For this review, take the finished solid that the model builds, in its own axes (mm). Face numbers are marked on the shaded views. Coordinates: 2 decimals unless noted, no trailing zeros. Write each loop counter-clockwise with the first axis right and the second up, starting at its lowest first coordinate (ties: lowest second). Pieces come first, ordered by that corner, then holes. Notation, with made-up numbers: (48, 51.25) -> (76, 51.25) arc R21 ccw to (76, 67.25) -> close; hole circle Ø3 at (-29, 24). An arc over 180 degrees is marked (long way). Put each result on its own line as item: value. Start each with the question number.
Item 1: To check wall thickness, follow L1, parallel to Y at x = 0, z = -4.45; L2, parallel to X at y = -0.5, z = -2.5; L3, parallel to Y at x = 2.25, z = -2.25. State the ranges of each line that lie inside material, in increasing order.
Item 2: Consider section A-A on z = 4.25. Give the boundary of the cut face in (x, y).
Item 3: The part is to be moulded in two halves that separate along Y. For the marked faces 1, 2 and 3, say which applies: +Y half, -Y half, draft (parallel to the pull), parting line (faces both ways), or undercut.
Item 4: Insertion check: P1, Ø1, axis at y = 1.5, z = -4.5, coming from the -X side; P2, Ø3, axis at x = 0, y = -3.5, coming from the +Z side; P3, Ø3, axis at x = -6, z = -2, coming from the +Y side; P4, Ø6, axis at x = 1, y = -2.5, coming from the -Z side. Each pin has a flat end and moves straight along its axis. Give the tip position at first contact, or say it passes through.
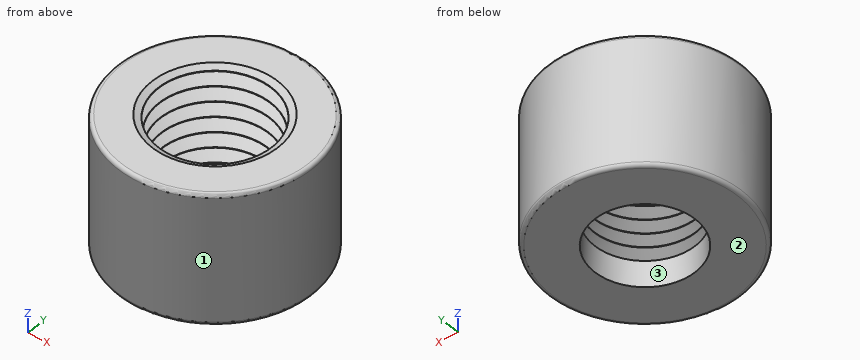
```python
from build123d import *

# Parameters (mm, degrees)
SKETCH1_R      = 9.398
EXTRUDE1_DEPTH = 6.35
SKETCH5_W      = 12.7
SKETCH5_H      = 4.869399387
FILLET1_R      = 0.352777778


with BuildPart() as part:
    # Sketch1 → Extrude1 (new body, symmetric)
    with BuildSketch(Plane.XY):
        Circle(SKETCH1_R)
    extrude(amount=EXTRUDE1_DEPTH, both=True)

    # Sketch5 → Cut-Revolve7 (revolve, cut)
    with BuildSketch(Plane(origin=(0, 0, 0), x_dir=(0, 0, -1), z_dir=(1, 0, 0))):
        with Locations((0, 2.434699694)):
            Rectangle(SKETCH5_W, SKETCH5_H)
    revolve(axis=Axis((0, 0, 0), (0, 0, -1)), mode=Mode.SUBTRACT)

    # Fillet1
    fillet1_edges = [part.edges().sort_by_distance(p)[0] for p in [
        (-9.398, 0, -6.35),
        (-9.398, 0, 6.35),
    ]]
    fillet(fillet1_edges, radius=FILLET1_R)

    # Sketch2 → Cut-Revolve5 (revolve, cut)
    with BuildSketch(Plane(origin=(0, 0, 0), x_dir=(0, 0, -1), z_dir=(1, 0, 0))):
        Polygon((-22.120436281, 7.622813225), (-21.540434076, 6.455429709), (-21.486747793, 6.452070868), (-20.765765115, 7.53805927), (-20.712078832, 7.534700429), (-20.132076627, 6.367316913), (-20.078390344, 6.363958072), (-19.357407666, 7.449946474), (-19.303721383, 7.446587633), (-18.723719178, 6.279204117), (-18.670032896, 6.275845277), (-17.949050217, 7.361833678), (-17.895363935, 7.358474838), (-17.31536173, 6.191091322), (-17.261675447, 6.187732481), (-16.540692769, 7.273720883), (-16.487006486, 7.270362042), (-15.907004281, 6.102978526), (-15.853317998, 6.099619685), (-15.13233532, 7.185608087), (-15.078649037, 7.182249246), (-14.498646832, 6.01486573), (-14.44496055, 6.01150689), (-13.723977871, 7.097495291), (-13.670291589, 7.094136451), (-13.090289384, 5.926752935), (-13.036603101, 5.923394094), (-12.315620423, 7.009382496), (-12.26193414, 7.006023655), (-11.681931935, 5.838640139), (-11.628245652, 5.835281298), (-10.907262974, 6.9212697), (-10.853576692, 6.917910859), (-10.273574486, 5.750527343), (-10.219888204, 5.747168503), (-9.498905526, 6.833156904), (-9.445219243, 6.829798064), (-8.865217038, 5.662414548), (-8.811530755, 5.659055707), (-8.090548077, 6.745044109), (-8.036861794, 6.741685268), (-7.456859589, 5.574301752), (-7.403173306, 5.570942911), (-6.682190628, 6.656931313), (-6.628504346, 6.653572472), (-6.04850214, 5.486188956), (-5.994815858, 5.482830116), (-5.27383318, 6.568818517), (-5.220146897, 6.565459677), (-4.640144692, 5.398076161), (-4.586458409, 5.39471732), (-3.865475731, 6.480705722), (-3.811789448, 6.477346881), (-3.231787243, 5.309963365), (-3.178100961, 5.306604524), (-2.457118282, 6.392592926), (-2.403432, 6.389234085), (-1.823429795, 5.221850569), (-1.769743512, 5.218491729), (-1.048760834, 6.30448013), (-0.995074551, 6.30112129), (-0.415072346, 5.133737774), (-0.361386063, 5.130378933), (0.359596615, 6.216367335), (0.413282898, 6.213008494), (0.993285103, 5.045624978), (1.046971385, 5.042266137), (1.767954064, 6.128254539), (1.821640346, 6.124895698), (2.401642551, 4.957512182), (2.455328834, 4.954153342), (3.176311512, 6.040141743), (3.229997795, 6.036782903), (3.81, 4.869399387), (3.81, 0), (-23.582480012, 0), (-23.582480012, 7.714284861), (-23.528793729, 7.71092602), (-22.948791524, 6.543542504), (-22.895105242, 6.540183664), (-22.174122563, 7.626172065), align=None)
    revolve(axis=Axis((0, 0, -97.9740637), (0, 0, 1)), mode=Mode.SUBTRACT)


solid = part.part
```
Return value:
1. L1: -9.4 to -4.87, 4.87 to 9.4
1. L2: -9.38 to -5, 5 to 9.38
1. L3: -9.12 to -4.76, 4.76 to 9.12
2. outline: circle Ø18.8 at (0, 0); hole circle Ø11.8 at (0, 0)
3. face 1: parting line
3. face 2: draft
3. face 3: undercut
4. P1: x = -9.34
4. P2: z = -2.38
4. P3: y = 8.25
4. P4: z = -6.35
